Can you work these out from the model? Positions are in its coordinate system, mm. A direction names the side the tool comes from. Give positions to 0.01 mm unless a question says otherwise; leave off trailing zeros. Loops run counter-clockwise (first coordinate to the right, second up) from the corner with the lowest first, then second, coordinate; pieces in that order, holes last. Notation, with made-up numbers: (35, -19) -> (76, -19) arc R21 ccw to (76, 12) -> close; hole circle Ø8 at (-19, 74). An arc over 180 degrees is marked (long way). One line per question, with ' | ' between items.
Autodesk Inventor part; units mm, degrees
ref_plane "YZ Plane" through (0, 0, 0) normal (1, 0, 0) x (0, 1, 0)
ref_plane "XZ Plane" through (0, 0, 0) normal (0, 1, 0) x (-1, 0, 0)
ref_plane "XY Plane" through (0, 0, 0) normal (0, 0, 1) x (1, 0, 0)
sketch "Sketch1" plane through (0, 0, 0) normal (0, 0, 1) x (1, 0, 0)
  circle A0 centre (0, 0) radius 10.5
  circle A1 centre (0, 0) radius 6
  dimension "d0" = 12
  dimension "d1" = 21
extrude "Extrusion1" add sketch "Sketch1" along normal blind 30
sketch "Sketch2" plane through (0, 0, 30) normal (0, 0, 1) x (1, 0, 0)
  circle A0 centre (0, 0) radius 6
  circle A1 centre (0, 0) radius 10.5
  line L0 (-15, -15) -> (15, -15)
  line L1 (15, -15) -> (15, 15)
  line L2 (15, 15) -> (-15, 15)
  line L3 (-15, 15) -> (-15, -15)
  line L4 (-15, -15) -> (15, 15) construction
  line L5 (15, -15) -> (-15, 15) construction
  dimension "d4" = 30
extrude "Extrusion2" add sketch "Sketch2" against normal blind 5 contours L3 L2 L1 L0
chamfer "Chamfer1" distance 2 angle 45 4 edges at (-15, 15, 27.5) (-15, -15, 27.5) (15, -15, 27.5) (15, 15, 27.5)
sketch "Sketch3" plane through (0, 0, 30) normal (0, 0, 1) x (1, 0, 0)
  point P0 (0, 0)
  point P1 (11.5, 11.5)
  point P2 (11.5, -11.5)
  point P3 (-11.5, -11.5)
  point P4 (-11.5, 11.5)
  dimension "d10" = 23
  dimension "d11" = 11.5
  dimension "d12" = 11.5
  dimension "d13" = 23
hole "Hole1" at (11.5, 11.5, 30) at (11.5, -11.5, 30) at (-11.5, -11.5, 30) at (-11.5, 11.5, 30) direction (0, 0, -1) diameter 3 depth 8 tip angle 118 counterbore diameter 6 counterbore depth 4
properties part number "LM12UU" material "Stainless Steel"
Q1. If we section it at C-C (y = 0): Write out the boundary of the cut face in (x, z).
Entries:
outline: (-15, 25) -> (-10.5, 25) -> (-10.5, 0) -> (-6, 0) -> (-6, 30) -> (-15, 30) -> close; (6, 0) -> (10.5, 0) -> (10.5, 25) -> (15, 25) -> (15, 30) -> (6, 30) -> close
Q2. If we section it at D-D (x = -4): Write out the boundary of the cut face in (y, z).
Entries:
outline: (-15, 25) -> (-9.71, 25) -> (-9.71, 0) -> (-4.47, 0) -> (-4.47, 30) -> (-15, 30) -> close; (4.47, 0) -> (9.71, 0) -> (9.71, 25) -> (15, 25) -> (15, 30) -> (4.47, 30) -> close
Q3. On a 3-axis mill with a long thin cutter (end or side, diameter ignored), from which of +Z, -Z, +X, -X, +Y, -Y can I reach the whole of each face in a straight line? I mean faces 1 (the face through (-14, -14, 28)), 2 (the face through (-9.7, 13.9, 28)), 3 (the face through (10, -3.2, 12.3)). Say none if no direction works.
Entries:
face 1: +Z, -Z, -X, -Y | face 2: +Z | face 3: -Z
Q4. For pin 1 Ø9.5 at (x, y) = (-11.5, -11.5) entering from -Z; pin 2 Ø4 at (x, y) = (-11.5, 11.5) entering from +Z; pin 3 Ø1.5 at (x, z) = (5.5, 18) entering from -Y, each with a flat end and sliding along its axis, tell me the tip position at first contact or that it passes through.
Entries:
pin 1: z = 25 | pin 2: z = 26 | pin 3: y = -9.36
Q5. If we section it at A-A (y = -11.5): Write out the boundary of the cut face in (x, z), plus the area to 3 significant figures.
Entries:
outline: (-15, 25) -> (-13, 25) -> (-13, 26) -> (-14.5, 26) -> (-14.5, 30) -> (-15, 30) -> close; (-10, 25) -> (10, 25) -> (10, 26) -> (8.5, 26) -> (8.5, 30) -> (-8.5, 30) -> (-8.5, 26) -> (-10, 26) -> close; (13, 25) -> (15, 25) -> (15, 30) -> (14.5, 30) -> (14.5, 26) -> (13, 26) -> close | area: 96.0 mm²
Q6. If we mould it in two halves opening along Y, with no side actions, what happens to faces 4 (the face through (0, 15, 28)), 5 (the face through (5, -5, 0)), 6 (the face through (-9.7, -9.1, 28))? For each: pulls with the +Y half, pulls with the -Y half, needs draft (parallel to the pull), parting line crosses it, or undercut.
Entries:
face 4: pulls with the +Y half | face 5: needs draft | face 6: undercut
Q7. If I drill on probe 1 along X at (y, z) = (11.5, 25.45); probe 2 along X at (y, z) = (-11.5, 28.85), over which ranges is the centre line in solid material (lowest first)? Write a range as from..to.
Entries:
probe 1: -15..-13, -10..10, 13..15 | probe 2: -15..-14.5, -8.5..8.5, 14.5..15
